CAD build for the part. Positions are in the model's coordinates, mm. A direction names the side the tool comes from. Coordinates: 2 decimals unless noted, no trailing zeros. Loops run counter-clockwise (first coordinate to the right, second up) from the corner with the lowest first, then second, coordinate; pieces in that order, holes last.
1) Saw through at C-C, the plane z = 42.5. Write the cut outline in (x, y).
2) Saw through at B-B, the plane x = 0. Write the cut outline in (y, z) (3 decimals), and give its area (3 significant figures).
3) Two-plate mould, pull along Z, no slides. Class faces 1 (the cylindrical face through (0.121, -37.465, -45.247)), 2 (the flat face through (-88, -38, 30)), 3 (the flat face through (-100, -38, 0)): +Z half, -Z half, draft (parallel to the pull), parting line (faces both ways), or undercut.
4) Saw through at D-D, the plane y = -21. Write the cut outline in (x, z).
5) Which spindle directions (+Z, -Z, +X, -X, +Y, -Y) get a long thin tool onto all of the face, cutting with end or side? Do faces 4 (the flat face through (-75, -38, -43)), 5 (the flat face through (88, -38, -30)), 6 (the flat face through (87, -38, 30)). Say none if no direction does.
6) Wall check: line 1 along Y through (x, z) = (66, -48.5); line 2 along X through (y, z) = (-38, 42); line 3 along X through (y, z) = (-1.5, 13). Give the ranges that are in metal, low to high.
7) Pin check, flat tips, straight feed: pin 1 Ø5 at (x, z) = (65.5, -20) entering from +Y; pin 2 Ø2.5 at (x, y) = (83.5, -36.5) entering from -Z; pin 3 Ø5.5 at (y, z) = (-37.5, 40.5) entering from +X; pin 4 Ø6 at (x, y) = (39, -28) entering from +Z. Stop position of each tip, or through.
8) Saw through at A-A, the plane z = 0. Write the cut outline in (x, y) (3 decimals).
```python
from build123d import *

# Parameters (mm, degrees)
SKETCH1_R           = 39.125
BOSS_EXTRUDE1_DEPTH = 8.75
SKETCH4_R           = 31.083201595
CUT_EXTRUDE1_DEPTH  = 9
BOSS_EXTRUDE3_START = 40
SKETCH5_R           = 35
SKETCH5_R_2         = 31.083201595
BOSS_EXTRUDE3_DEPTH = 40
SKETCH8_R           = 50
BOSS_EXTRUDE4_DEPTH = 5
SKETCH10_R          = 2.75
CUT_EXTRUDE2_DEPTH  = 5
CUT_EXTRUDE3_START  = -5
SKETCH11_R          = 31.083201595
CUT_EXTRUDE3_DEPTH  = 5
SKETCH12_R          = 2.75
SKETCH12_R_2        = 31.083201595
BOSS_EXTRUDE5_DEPTH = 5
FILLET2_R           = 4


with BuildPart() as part:
    # Sketch1 → Boss-Extrude1 (new body)
    with BuildSketch(Plane(origin=(0, 0, 0), x_dir=(1, 0, 0), z_dir=(0, 1, 0))):
        with Locations(Location((0, 0, 0), (0, 0, 270))):
            Circle(SKETCH1_R)
    extrude(amount=BOSS_EXTRUDE1_DEPTH)

    # Sketch4 → Cut-Extrude1 (cut)
    with BuildSketch(Plane.XZ):
        with Locations(Location((0, 0, 0), (0, 0, 270))):
            Circle(SKETCH4_R)
    extrude(amount=-CUT_EXTRUDE1_DEPTH, mode=Mode.SUBTRACT)

    # Sketch5 → Boss-Extrude3 (add)
    with BuildSketch(Plane.XZ.offset(BOSS_EXTRUDE3_START)):
        with Locations(Location((0, 0, 0), (0, 0, 270))):
            Circle(SKETCH5_R)
        with Locations(Location((0, 0, 0), (0, 0, 270))):
            Circle(SKETCH5_R_2, mode=Mode.SUBTRACT)
    extrude(amount=-BOSS_EXTRUDE3_DEPTH)

    # Sketch8 → Boss-Extrude4 (add)
    with BuildSketch(Plane.XZ.offset(40)):
        with Locations(Location((0, 0, 0), (0, 0, 270))):
            Circle(SKETCH8_R)
    extrude(amount=-BOSS_EXTRUDE4_DEPTH)

    # Sketch10 → Cut-Extrude2 (cut)
    with BuildSketch(Plane(origin=(0, -35, 0), x_dir=(1, 0, 0), z_dir=(0, 1, 0))):
        with Locations(Location((0, 42.5, 0), (0, 0, 270))):
            Circle(SKETCH10_R)
        with Locations(Location((42.5, 0, 0), (0, 0, 270))):
            Circle(SKETCH10_R)
        with Locations(Location((0, -42.5, 0), (0, 0, 270))):
            Circle(SKETCH10_R)
        with Locations(Location((-42.5, 0, 0), (0, 0, 270))):
            Circle(SKETCH10_R)
    extrude(amount=-CUT_EXTRUDE2_DEPTH, mode=Mode.SUBTRACT)

    # Sketch11 → Cut-Extrude3 (cut)
    with BuildSketch(Plane(origin=(0, -35, 0), x_dir=(1, 0, 0), z_dir=(0, 1, 0)).offset(CUT_EXTRUDE3_START)):
        with Locations(Location((0, 0, 0), (0, 0, 270))):
            Circle(SKETCH11_R)
    extrude(amount=CUT_EXTRUDE3_DEPTH, mode=Mode.SUBTRACT)

    # Sketch12 → Boss-Extrude5 (add)
    with BuildSketch(Plane.XZ.offset(40)):
        Polygon((-75, 55), (75, 55), (75, 30), (100, 30), (100, -30), (75, -30), (75, -55), (-75, -55), (-75, -30), (-100, -30), (-100, 30), (-75, 30), align=None)
        with Locations(Location((0, 42.5, 0), (0, 0, 90))):
            Circle(SKETCH12_R, mode=Mode.SUBTRACT)
        with Locations(Location((0, -42.5, 0), (0, 0, 90))):
            Circle(SKETCH12_R, mode=Mode.SUBTRACT)
        with Locations(Location((0, 0, 0), (0, 0, 90))):
            Circle(SKETCH12_R_2, mode=Mode.SUBTRACT)
    extrude(amount=-BOSS_EXTRUDE5_DEPTH)

    # Fillet2
    fillet2_edges = [part.edges().sort_by_distance(p)[0] for p in [
        (0, -35, 35),
    ]]
    fillet(fillet2_edges, radius=FILLET2_R)


solid = part.part
```
Data:
1. outline: (-75, -40) - (-2.75, -40) - (-2.75, -35) - (-75, -35) - close; (2.75, -40) - (75, -40) - (75, -35) - (2.75, -35) - close
2. outline: (-40, -55) - (-35, -55) - (-35, -45.25) - (-40, -45.25) - close; (-40, -39.75) - (-35, -39.75) - (-35, -39) arc R4 cw to (-31, -35) - (0, -35) - (0, -39.125) - (8.75, -39.125) - (8.75, -31.083) - (-40, -31.083) - close; (-40, 31.083) - (8.75, 31.083) - (8.75, 39.125) - (0, 39.125) - (0, 35) - (-31, 35) arc R4 cw to (-35, 39) - (-35, 39.75) - (-40, 39.75) - close; (-40, 45.25) - (-35, 45.25) - (-35, 55) - (-40, 55) - close
2. area: 606 mm2
3. face 1: undercut
3. face 2: +Z half
3. face 3: draft
4. outline: circle Ø70 at (0, 0); hole circle Ø62.17 at (0, 0)
5. face 4: -Z, -X, +Y, -Y
5. face 5: -Z, +X, +Y, -Y
5. face 6: +Z, +X, +Y, -Y
6. line 1: y = -40 to -35
6. line 2: x = -75 to -2.7, 2.7 to 75
6. line 3: x = -32.5 to -28.23, 28.23 to 32.5
7. pin 1: stops at y = -35
7. pin 2: stops at z = -30
7. pin 3: stops at x = 75
7. pin 4: passes through
8. outline: (-100, -40) - (-31.083, -40) - (-31.083, 8.75) - (-39.125, 8.75) - (-39.125, 0) - (-35, 0) - (-35, -31) arc R4 cw to (-39, -35) - (-100, -35) - close; (31.083, -40) - (100, -40) - (100, -35) - (39, -35) arc R4 cw to (35, -31) - (35, 0) - (39.125, 0) - (39.125, 8.75) - (31.083, 8.75) - close
